CAD build for the part. Positions are in the model's coordinates, mm. Round coordinates to 2 decimals unless told otherwise and drop trailing zeros. Loops run counter-clockwise (first coordinate to the right, second up) from the corner with the lowest first, then second, coordinate; pieces in that order, holes last. Notation, with made-up numbers: M 9.5,42.25 L 28.5,42.25 A12 cw 28.5,47.25 Z; hole C 45.25,-22 d8. An arc over 180 degrees is marked long. Use a Markdown table: item, result. Add a question column.
(1) Two-plate mould, pull along Y, no slides. Class faces 1 (the face through (-15.64, 7.87, 1.61)), 2 (the face through (-15.273, -9.666, 1.565)), 3 (the face through (10, -10, 3.175)), 4 (the face through (-18.267, -14.007, 1.565)): released by +Y, released by -Y, zero draft, split by the parting line, or undercut.
(2) Band-saw the part on D-D, the plane z = 0.75. Give the number of separate pieces and of enclosed holes in the cut face, and give its area (3 significant figures).
(3) Wall check: L1, parallel to Y at x = 0.5, z = 1.4; L2, parallel to Y at x = -12.5, z = 1.5; L3, parallel to X at y = -3.5, z = 2.3. Give the ranges that are in metal, low to high.
(4) Band-saw the part on A-A, the plane y = 0. Write the cut outline in (x, z) (3 decimals), and give its area (3 significant figures).
(5) Band-saw the part on C-C, the plane y = -19. Write the cut outline in (x, z) (3 decimals), and give its area (3 significant figures).
(6) Flat gauge pins, fed straight in: P1, Ø5, axis at x = -12.35, y = -12.35, coming from the -Z side; P2, Ø1.5, axis at y = 1, z = 0.5, coming from the +X side. Where does each tip first touch, or does it go through?
from build123d import *

# Parameters (mm, degrees)
F0_R     = 23.01875
F0_R_2   = 3.96875
F0_R_3   = 2.15265
F0_R_4   = 11.90625
F1_DEPTH = 3.175
F3_DEPTH = 3.175


with BuildPart() as f1:
    # F0 (on Top) → F1 (new body)
    with BuildSketch(Plane.XY):
        Circle(F0_R)
        with Locations((-12.347852, -12.347852)):
            Circle(F0_R_2, mode=Mode.SUBTRACT)
        with Locations((12.347852, -12.347852)):
            Circle(F0_R_3, mode=Mode.SUBTRACT)
        with Locations((-12.347852, 12.347852)):
            Circle(F0_R_3, mode=Mode.SUBTRACT)
        Circle(F0_R_4, mode=Mode.SUBTRACT)
        with Locations((12.347852, 12.347852)):
            Circle(F0_R_2, mode=Mode.SUBTRACT)
    extrude(amount=F1_DEPTH)

    # F2 (on face) → F3 (cut, through all)
    with BuildSketch(Plane.XY.offset(3.175)):
        with BuildLine():
            ThreePointArc((-9.771912, 17.270905), (-7.8939, 15.669632), (-6.894649, 13.412976))
            ThreePointArc((-6.894649, 13.412976), (0, 15.08125), (6.894649, 13.412976))
            ThreePointArc((6.894649, 13.412976), (7.8939, 15.669632), (9.771912, 17.270905))
            ThreePointArc((9.771912, 17.270905), (0, 19.84375), (-9.771912, 17.270905))
        make_face()
        with BuildLine():
            ThreePointArc((-13.412976, 6.894649), (-15.669632, 7.8939), (-17.270905, 9.771912))
            ThreePointArc((-17.270905, 9.771912), (-19.84375, 0), (-17.270905, -9.771912))
            ThreePointArc((-17.270905, -9.771912), (-15.669632, -7.8939), (-13.412976, -6.894649))
            ThreePointArc((-13.412976, -6.894649), (-15.08125, 0), (-13.412976, 6.894649))
        make_face()
        with BuildLine():
            ThreePointArc((17.270905, 9.771912), (15.669632, 7.8939), (13.412976, 6.894649))
            ThreePointArc((13.412976, 6.894649), (15.08125, 0), (13.412976, -6.894649))
            ThreePointArc((13.412976, -6.894649), (15.669632, -7.8939), (17.270905, -9.771912))
            ThreePointArc((17.270905, -9.771912), (19.84375, 0), (17.270905, 9.771912))
        make_face()
        with BuildLine():
            ThreePointArc((-6.894649, -13.412976), (-7.8939, -15.669632), (-9.771912, -17.270905))
            ThreePointArc((-9.771912, -17.270905), (0, -19.84375), (9.771912, -17.270905))
            ThreePointArc((9.771912, -17.270905), (7.8939, -15.669632), (6.894649, -13.412976))
            ThreePointArc((6.894649, -13.412976), (0, -15.08125), (-6.894649, -13.412976))
        make_face()
    extrude(amount=-F3_DEPTH, mode=Mode.SUBTRACT)


solid = f1.part
Return value:
| question | item | result |
|---|---|---|
| 1 | face 1 | undercut |
| 1 | face 2 | undercut |
| 1 | face 3 | zero draft |
| 1 | face 4 | split by the parting line |
| 2 | separate pieces | 1 |
| 2 | enclosed holes | 9 |
| 2 | area | 774 mm^2 |
| 3 | L1 | -23.01 to -19.84, -15.07 to -11.9, 11.9 to 15.07, 19.84 to 23.01 |
| 3 | L2 | -19.33 to -16.31, -8.38 to 10.2, 14.5 to 19.33 |
| 3 | L3 | -22.75 to -19.53, -14.67 to -11.38, 11.38 to 14.67, 19.53 to 22.75 |
| 4 | outline | M -23.019,0 L -19.844,0 L -19.844,3.175 L -23.019,3.175 Z; M -15.081,0 L -11.906,0 L -11.906,3.175 L -15.081,3.175 Z; M 11.906,0 L 15.081,0 L 15.081,3.175 L 11.906,3.175 Z; M 19.844,0 L 23.019,0 L 23.019,3.175 L 19.844,3.175 Z |
| 4 | area | 40.3 mm^2 |
| 5 | outline | M -12.995,0 L -5.725,0 L -5.725,3.175 L -12.995,3.175 Z; M 5.725,0 L 12.995,0 L 12.995,3.175 L 5.725,3.175 Z |
| 5 | area | 46.2 mm^2 |
| 6 | P1 | through |
| 6 | P2 | x = 23.02 |
